Read the model definition and answer for the solid it produces. Units are mm, in the model's axes. Give positions to 0.01 mm unless a question says otherwise; leave off trailing zeros. Loops run counter-clockwise (first coordinate to the right, second up) from the corner with the lowest first, then second, coordinate; pieces in that order, holes last. Notation, with made-up numbers: (74.25, -37) - (105.25, -37) arc R17 cw to (105.25, -28) - close; hole circle Ø10 at (-25, 39). An arc over 180 degrees is marked (long way). Use a Markdown table: item, result. Add a question column.
Item 1: Consider probe 1 along X at (y, z) = (-3.8, 8.75); probe 2 along X at (y, z) = (-3.45, 6.5); probe 3 along Z at (x, y) = (33.5, -3.5). Determine where each line is inside the solid, lowest interval first. Write a range as [from, to].
Item 2: A cutting plane is placed at B-B (y = -1.2). Determine the outline of the cut face in (x, z), plus the area to 3 significant figures.
Item 3: A cutting plane is placed at A-A (x = 35.5). Determine the outline of the cut face in (y, z).
from build123d import *

# Parameters (mm, degrees)
F0_W     = 40
F0_H     = 25
F1_DEPTH = 4
F2_SIZE  = 1
F3_SIZE  = 2


with BuildPart() as f1:
    # F0 (on Front) → F1 (new body)
    with BuildSketch(Plane.XZ):
        with Locations((20, 12.5)):
            Rectangle(F0_W, F0_H)
    extrude(amount=F1_DEPTH)

    # F2
    f2_edges = [f1.edges().sort_by_distance(p)[0] for p in [
        (0, -4, 12.5),
        (20, -4, 0),
        (40, -4, 12.5),
    ]]
    chamfer(f2_edges, length=F2_SIZE)

    # F3
    f3_edges = [f1.edges().sort_by_distance(p)[0] for p in [
        (20, 0, 25),
    ]]
    chamfer(f3_edges, length=F3_SIZE)


solid = f1.part
Geometry says:
| question | item | result |
|---|---|---|
| 1 | probe 1 | [0.8, 39.2] |
| 1 | probe 2 | [0.45, 39.55] |
| 1 | probe 3 | [0.5, 25] |
| 2 | outline | (0, 0) - (40, 0) - (40, 24.2) - (0, 24.2) - close |
| 2 | area | 968 mm² |
| 3 | outline | (-4, 1) - (-3, 0) - (0, 0) - (0, 23) - (-2, 25) - (-4, 25) - close |
